Verification items for this drawing (mm, ordinates from the low corner). A direction names the side the tool comes from. Round coordinates to 2 decimals unless told otherwise and drop trailing zeros. Loops run counter-clockwise (first coordinate to the right, second up) from the corner with the lowest first, then second, coordinate; pieces in that order, holes last. Notation, with made-up numbers: (-3, 9.25) -> (28, 9.25) arc R12 ccw to (28, 19.25) -> close; hole circle Ø11 at (76.25, 74.25). An arc over 180 degrees is marked (long way). One line per question, with ' | ' between items.
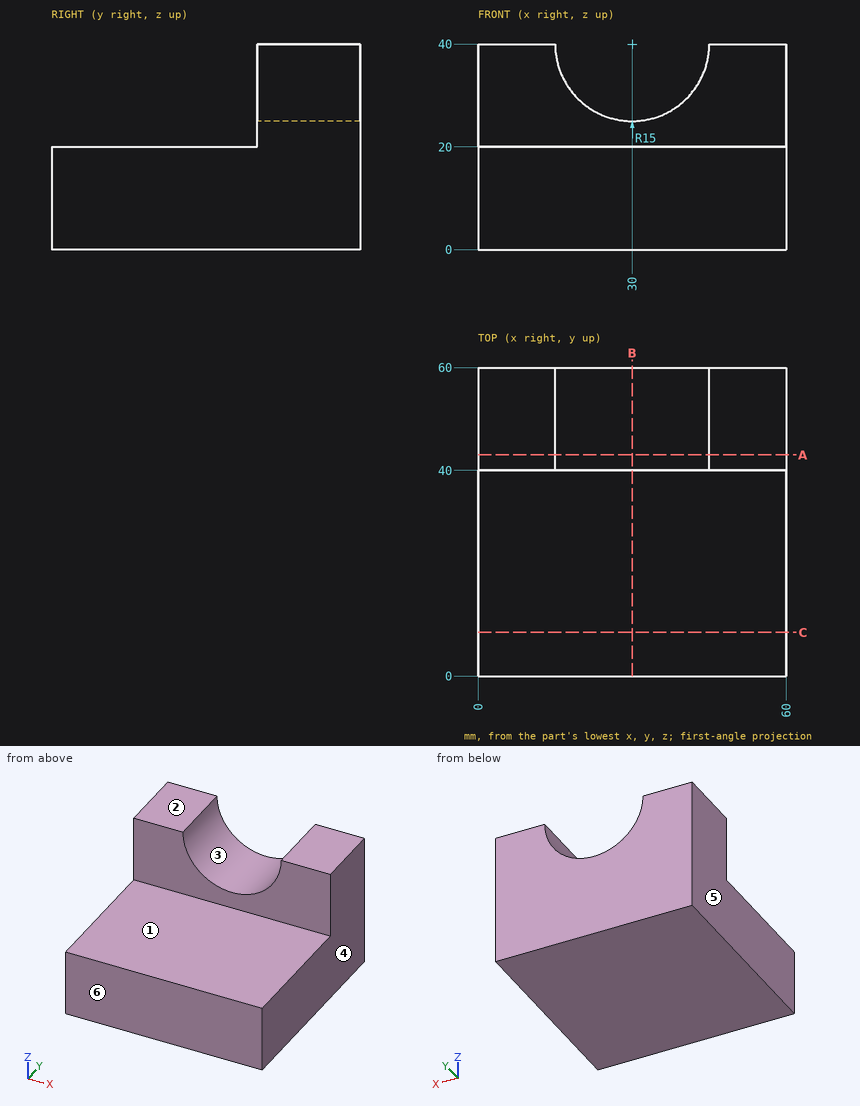
(1) Mould release check, pull along X, two halves, no side actions. Record for the marked faces 3, 4, 5 and 6: +X half, -X half, draft (parallel to the pull), parting line (faces both ways), or undercut.
Answer:
face 3: undercut | face 4: +X half | face 5: -X half | face 6: draft
(2) Sectioned sample at B-B, the plane x = 30. Record the cut outline in (y, z), and give its area (3 significant figures).
Answer:
outline: (0, 0) -> (60, 0) -> (60, 25) -> (40, 25) -> (40, 20) -> (0, 20) -> close | area: 1,300 mm2
(3) Sectioned sample at A-A, the plane y = 43. Record the cut outline in (x, z).
Answer:
outline: (0, 0) -> (60, 0) -> (60, 40) -> (45, 40) arc R15 cw to (15, 40) -> (0, 40) -> close
(4) Set-up check for the marked faces 1 and 2: record each of +Z, -Z, +X, -X, +Y, -Y from which the full face is reachable in a straight line by a thin tool's end or side.
Answer:
face 1: +Z, +X, -X, -Y | face 2: +Z, +X, -X, +Y, -Y
(5) Go/stop test with flat-tipped pins: pin 1 (10 mm diameter, centred on x = 52, y = 33.5, fed in from +Z); pin 2 (16 mm diameter, centred on x = 28, z = 29, fed in from -Y). Record where each tip stops, or that it passes through.
Answer:
pin 1: stops at z = 20 | pin 2: stops at y = 40
(6) Scan lines: probe 1 along Z at (x, y) = (25, 16); probe 2 along X at (y, z) = (44.5, 35.5); probe 3 along Y at (x, z) = (4, 21.5). Record each from-to range of solid material in increasing order.
Answer:
probe 1: z = 0 to 20 | probe 2: x = 0 to 15.69, 44.31 to 60 | probe 3: y = 40 to 60
(7) Sectioned sample at C-C, the plane y = 8.5. Record the cut outline in (x, z), and give its area (3 significant figures).
Answer:
outline: (0, 0) -> (60, 0) -> (60, 20) -> (0, 20) -> close | area: 1,200 mm2
